```python
from build123d import *


with BuildPart() as part:
    # Sketch1 → Revolve-Thin1 (revolve)
    with BuildSketch(Plane.XY):
        Polygon((286.093493363, 15), (204.063493363, 15), (204.063493363, 20), (171.093493363, 20), (171.093493363, 15), (116.093493363, 15), (116.093493363, 20), (83.123493363, 20), (83.123493363, 15), (10.153493363, 15), (10.153493363, 20), (-22.816506637, 20), (-22.816506637, 15), (-143.276508184, 15), (-374.696506637, 15), (-374.696506637, 5), (-143.276508184, 5), (-12.816506637, 5), (-12.816506637, 10), (0.153493363, 10), (0.153493363, 5), (93.123493363, 5), (93.123493363, 10), (106.093493363, 10), (106.093493363, 5), (181.093493363, 5), (181.093493363, 10), (194.063493363, 10), (194.063493363, 5), (286.093493363, 5), align=None)
    revolve(axis=Axis((-141.82946491, 0, 0), (1, 0, 0)))


solid = part.part
```
CAD build for the part. Positions are in the model's coordinates, mm. A direction names the side the tool comes from. Coordinates: 2 decimals unless noted, no trailing zeros. Order: outer loops, then holes, each group sorted by start corner. A loop starts at its lowest first (then second) coordinate and runs counter-clockwise, first axis right, second up. Notation, with made-up numbers: (54.5, -39.5) -> (74.5, -39.5) arc R13 cw to (74.5, -34.5) -> close; hole circle Ø10 at (-30, -5.75). An arc over 180 degrees is marked (long way). Use one line per item in the form item = value. Start each with the question number.
1) Tool access for faces 1 (the flat face through (181.093, -2, 5)), 2 (the cylindrical face through (-191.22, -1.08, -4.88)), 3 (the cylindrical face through (-201.22, -14.985, 0.66)), 4 (the cylindrical face through (244.504, -14.985, 0.66)): list every direction of +Z, -Z, +X, -X, +Y, -Y with a clear straight run to the whole face (end or side of a thin tool).
2) Pull direction X, two halves, no side cores. Call faces 5 (the cylindrical face through (240.72, -1.08, -4.88)), 6 (the flat face through (10.153, -3, 15)), 7 (the flat face through (-374.697, -4, 4)): +X half, -X half, draft (parallel to the pull), parting line (faces both ways), or undercut.
3) Drill centre lines: L1, parallel to X at y = 2.5, z = 8; L2, parallel to X at y = -15, z = 1.5; L3, parallel to Z at x = -258, y = 0. Where is each one in solid material? Low to high. Write a range as [from, to].
4) Band-saw the part on A-A on x = 161.5. Give the cut face in (y, z).
5) Drop flat-ended pins along their axis: pin 1 (8 mm diameter, centred on x = 94, y = -5, fed in from -Z) (3 decimals); pin 2 (5 mm diameter, centred on x = -77.5, y = 6.5, fed in from -Z); pin 3 (12 mm diameter, centred on x = -51.5, z = 0, fed in from -Y). Give the stop position or say it passes through.
Entries:
q1.face_1 = none
q1.face_2 = +X, -X
q1.face_3 = -X
q1.face_4 = +X
q2.face_5 = draft
q2.face_6 = undercut
q2.face_7 = -X half
q3.L1 = [-374.7, -12.82], [0.15, 93.12], [106.09, 181.09], [194.06, 286.09]
q3.L2 = [-22.82, 10.15], [83.12, 116.09], [171.09, 204.06]
q3.L3 = [-15, -5], [5, 15]
q4.outline = circle Ø30 at (0, 0); hole circle Ø10 at (0, 0)
q5.pin_1 = -19.975
q5.pin_2 = -14.46
q5.pin_3 = -15
